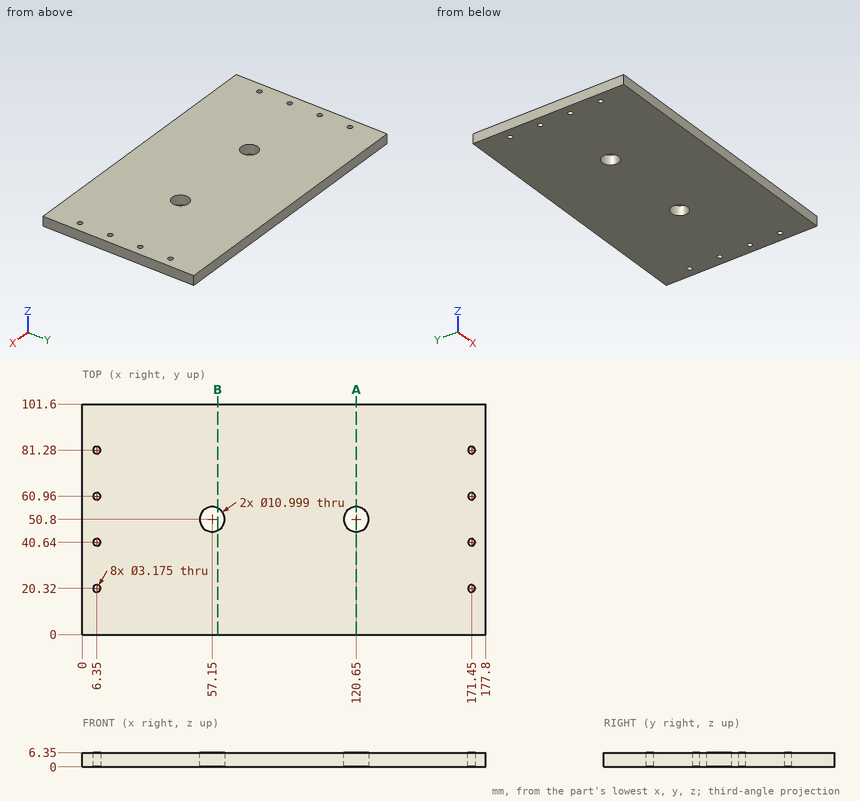
Geometry check sheet. Reference: drawing and pictorial views, mm from the part's lowest x, y, z. Coordinates: 2 decimals unless noted, no trailing zeros. Order: outer loops, then holes, each group sorted by start corner. A loop starts at its lowest first (then second) coordinate and runs counter-clockwise, first axis right, second up.
Item 1: Section check A-A, the plane x = 120.65. Enter the section's corners in (y, z).
Filled in:
outline: (0, 0) - (45.3, 0) - (45.3, 6.35) - (0, 6.35) - close; (56.3, 0) - (101.6, 0) - (101.6, 6.35) - (56.3, 6.35) - close
Item 2: Section check B-B, the plane x = 59.5. Enter the section's corners in (y, z), then the cut area to 3 significant figures.
Filled in:
outline: (0, 0) - (45.83, 0) - (45.83, 6.35) - (0, 6.35) - close; (55.77, 0) - (101.6, 0) - (101.6, 6.35) - (55.77, 6.35) - close
area: 582 mm2
Item 3: Material ranges on L1, parallel to Y at x = 6.35, z = 5.25; L2, parallel to Y at x = 120.65, z = 1.75; L3, parallel to X at y = 52, z = 5, recorded low to high.
Filled in:
L1: y = 0 to 18.73, 21.91 to 39.05, 42.23 to 59.37, 62.55 to 79.69, 82.87 to 101.6
L2: y = 0 to 45.3, 56.3 to 101.6
L3: x = 0 to 51.78, 62.52 to 115.28, 126.02 to 177.8
